Autodesk Inventor part; units mm, degrees
ref_plane "工作平面2" through (150, 0, 0) normal (-1, 0, 0) x (0, 0, 1)
ref_plane "YZ Plane" through (0, 0, 0) normal (1, 0, 0) x (0, 1, 0)
ref_plane "XZ Plane" through (0, 0, 0) normal (0, 1, 0) x (-1, 0, 0)
sketch "草圖1" plane through (0, 0, 0) normal (0, 0, 1) x (1, 0, 0)
  line L0 (0, 25) -> (300, 25)
  line L1 (300, 25) -> (300, 0)
  line L2 (300, 0) -> (0, 0)
  line L3 (0, 0) -> (0, 25)
  circle A0 centre (23, 17.5) radius 6.55
  circle A1 centre (277, 17.5) radius 2
  line L4 (16, 0) -> (24, 0)
  line L5 (24, 0) -> (24, -2.9)
  line L6 (24, -2.9) -> (16, -2.9)
  line L7 (16, -2.9) -> (16, 0)
  line L8 (276, 0) -> (284, 0)
  line L9 (284, 0) -> (284, -2.9)
  line L10 (284, -2.9) -> (276, -2.9)
  line L11 (276, -2.9) -> (276, 0)
  line L12 (0, 25) -> (5, 25)
  line L13 (5, 25) -> (5, 0)
  line L14 (5, 0) -> (0, 0)
  line L15 (0, 0) -> (0, 25)
  line L16 (300, 25) -> (295, 25)
  line L17 (295, 25) -> (295, 0)
  line L18 (295, 0) -> (300, 0)
  line L19 (300, 0) -> (300, 25)
  line L20 (24, -1.45) -> (276, -1.45) construction
  point P0 (16, -1.45)
  point P1 (284, -1.45)
  point P2 (284, 0)
  point P3 (24, 0)
  point P4 (150, -1.45)
  point P5 (150, 0)
  dimension "d0" = 300
  dimension "d1" = 25
  dimension "d2" = 7.5
  dimension "d3" = 13.1
  dimension "d4" = 23
  dimension "d5" = 23
  dimension "d6" = 7.5
  dimension "d7" = 4
  dimension "d12" = 8
  dimension "d13" = 2.9
  dimension "d14" = 8
  dimension "d30" = 5
  dimension "d31" = 5
  dimension "d32" = 252
extrude "擠出1" add sketch "草圖1" along normal blind 3 contours L0 L17 L2 L13 | L2 L5 L6 L7 | L9 L10 L11 L2
sketch "草圖2" plane through (0, 0, 3) normal (0, 0, 1) x (1, 0, 0)
  line L0 (10.5404, 25) -> (13.4864, 25.1544)
  line L1 (13.4864, 25.1544) -> (14.0097, 15.1681)
  line L2 (14.0097, 15.1681) -> (11.0638, 15.0137)
  line L3 (11.0638, 15.0137) -> (10.5404, 25)
  line L4 (295, 25) -> (5, 25)
  line L5 (16.048, 25) -> (29.13, 25.6856)
  line L6 (29.13, 25.6856) -> (30.1465, 6.2887)
  line L7 (30.1465, 6.2887) -> (17.0645, 5.6031)
  line L8 (17.0645, 5.6031) -> (16.048, 25)
  circle A0 centre (23, 17.5) radius 6.55
  line L9 (14.0097, 15.1681) -> (16.5562, 15.3016)
  line L10 (286.4135, 25.1544) -> (289.3595, 25)
  line L11 (289.3595, 25) -> (288.8361, 15.0137)
  line L12 (288.8361, 15.0137) -> (285.8901, 15.1681)
  line L13 (285.8901, 15.1681) -> (286.4135, 25.1544)
  line L14 (275.2453, 22.2337) -> (279.2399, 22.0243)
  line L15 (279.2399, 22.0243) -> (278.6818, 11.3762)
  line L16 (278.6818, 11.3762) -> (274.6873, 11.5855)
  line L17 (274.6873, 11.5855) -> (275.2453, 22.2337)
  circle A1 centre (277, 17.5) radius 2
  line L18 (285.8901, 15.1681) -> (278.8997, 15.5344)
  point P0 (0, 0)
  point P1 (300, 25)
  point P2 (0, 25)
  point P3 (286.4054, 25)
  point P4 (13.4945, 25)
  dimension "d16" = 2.95
  dimension "d18" = 10
  dimension "d19" = 87
  dimension "d20" = 87
  dimension "d22" = 87
  dimension "d23" = 87
  dimension "d24" = 2.95
  dimension "d25" = 10
  dimension "d33" = 9.1
  dimension "d34" = 9
extrude "擠出2" cut sketch "草圖2" against normal up to surface (3 mm away) contours L4 L11 L12 L13 | L4 L1 L2 L3
sketch "草圖7" plane through (0, 0, 3) normal (0, 0, 1) x (1, 0, 0)
  line L0 (64.4714, 28.6858) -> (65.4135, 10.7104)
  line L1 (65.4135, 10.7104) -> (7.493, 7.675)
  line L2 (7.493, 7.675) -> (6.5509, 25.6503)
  line L3 (6.5509, 25.6503) -> (64.4714, 28.6858)
  line L4 (13.4945, 25) -> (14.0097, 15.1681)
  circle A0 centre (23, 17.5) radius 6.55
  line L5 (285.8901, 15.1681) -> (286.4054, 25)
  line L6 (286.4054, 25) -> (13.4945, 25)
  line L7 (13.4945, 25) -> (14.0097, 15.1681)
  line L8 (14.0097, 15.1681) -> (11.0638, 15.0137)
  line L9 (11.0638, 15.0137) -> (10.5404, 25)
  line L10 (10.5404, 25) -> (5, 25)
  line L11 (5, 25) -> (5, 0)
  line L12 (5, 0) -> (16, 0)
  line L13 (16, 0) -> (16, -2.9)
  line L14 (16, -2.9) -> (24, -2.9)
  line L15 (24, -2.9) -> (24, 0)
  line L16 (24, 0) -> (276, 0)
  line L17 (276, 0) -> (276, -2.9)
  line L18 (276, -2.9) -> (284, -2.9)
  line L19 (284, -2.9) -> (284, 0)
  line L20 (284, 0) -> (295, 0)
  line L21 (295, 0) -> (295, 25)
  line L22 (295, 25) -> (289.3595, 25)
  line L23 (289.3595, 25) -> (288.8361, 15.0137)
  line L24 (288.8361, 15.0137) -> (285.8901, 15.1681)
  circle A1 centre (23, 17.5) radius 6.55
  circle A2 centre (277, 17.5) radius 2
  line L25 (13.4945, 25) -> (13.4414, 26.0114)
  line L26 (10.5404, 25) -> (11.0638, 15.0137)
  line L27 (10.5404, 25) -> (10.4955, 25.857)
  point P0 (0, 0)
  point P1 (64.6646, 25)
  point P2 (6.585, 25)
  dimension "d50" = 42
  dimension "d51" = 16
  dimension "d52" = 18
  dimension "d53" = 9
extrude "擠出5" add sketch "草圖7" against normal up to surface (3 mm away) contours L0 L6 L25 L3 | L27 L10 L2 L3
sketch "草圖9" plane through (0, 0, 3) normal (0, 0, 1) x (1, 0, 0)
  line L0 (10.4955, 25.857) -> (6.5509, 25.6503)
  line L1 (6.5509, 25.6503) -> (64.4714, 28.6858)
  line L2 (64.4714, 28.6858) -> (65.4135, 10.7104)
  line L3 (65.4135, 10.7104) -> (7.493, 7.675)
  line L4 (7.493, 7.675) -> (6.5509, 25.6503)
  circle A0 centre (58.1897, 24.3511) radius 2
  circle A1 centre (58.713, 14.3648) radius 2
  line L5 (58.1897, 24.3511) -> (58.713, 14.3648)
  line L6 (58.4513, 19.3579) -> (64.9424, 19.6981)
  circle A2 centre (23, 17.5) radius 6.55
  point P0 (0, 0)
  dimension "d60" = 18
  dimension "d64" = 4
  dimension "d66" = 6.5
  dimension "d67" = 10
extrude "擠出6" cut sketch "草圖9" against normal up to surface (3 mm away) contours A1 | A0
sketch "草圖11" plane through (0, 0, 3) normal (0, 0, 1) x (1, 0, 0)
  line L0 (16.45, 26.8556) -> (29.55, 26.8556)
  line L1 (29.55, 26.8556) -> (29.55, 17.5)
  line L2 (29.55, 17.5) -> (16.45, 17.5)
  line L3 (16.45, 17.5) -> (16.45, 26.8556)
  circle A0 centre (23, 17.5) radius 6.55
  line L4 (64.4714, 28.6858) -> (13.4414, 26.0114)
  point P0 (0, 0)
  dimension "d74" = 13.1
extrude "擠出7" cut sketch "草圖11" against normal blind 10 contours L0 L4 L3 | L1 A0 L3 L4 | L2 A0 picked at (21.0033, 19.0372)
ref_plane "工作平面2" through (150, 0, 0) normal (-1, 0, 0) x (0, 0, 1)
mirror "鏡射2" [suppressed]
sketch "草圖12" plane through (0, 0, 3) normal (0, 0, 1) x (1, 0, 0)
  arc A0 (279, 17.5) -> (279, 17.5) centre (277, 17.5) ccw
  line L0 (279, 17.5) -> (283.55, 17.5)
  circle A1 centre (277, 17.5) radius 6.55
  point P0 (0, 0)
extrude "擠出8" [suppressed]
sketch "草圖10" plane through (0, 0, 3) normal (0, 0, 1) x (1, 0, 0)
  line L0 (285.8901, 15.1681) -> (286.4054, 25)
  line L1 (286.4054, 25) -> (64.6646, 25)
  line L2 (14.0097, 15.1681) -> (11.0638, 15.0137)
  line L3 (6.585, 25) -> (5, 25)
  line L4 (5, 25) -> (5, 0)
  line L5 (5, 0) -> (16, 0)
  line L6 (16, 0) -> (16, -2.9)
  line L7 (16, -2.9) -> (24, -2.9)
  line L8 (24, -2.9) -> (24, 0)
  line L9 (24, 0) -> (276, 0)
  line L10 (276, 0) -> (276, -2.9)
  line L11 (276, -2.9) -> (284, -2.9)
  line L12 (284, -2.9) -> (284, 0)
  line L13 (284, 0) -> (295, 0)
  line L14 (295, 0) -> (295, 25)
  line L15 (295, 25) -> (289.3595, 25)
  line L16 (289.3595, 25) -> (288.8361, 15.0137)
  line L17 (288.8361, 15.0137) -> (285.8901, 15.1681)
  arc A0 (16.45, 17.5) -> (29.55, 17.5) centre (23, 17.5) ccw
  circle A1 centre (277, 17.5) radius 2
  line L18 (13.4414, 26.0114) -> (14.0097, 15.1681)
  line L19 (11.0638, 15.0137) -> (10.4955, 25.857)
  line L20 (64.6646, 25) -> (64.4714, 28.6858)
  line L21 (64.4714, 28.6858) -> (29.55, 26.8556)
  line L22 (10.4955, 25.857) -> (6.5509, 25.6503)
  line L23 (6.5509, 25.6503) -> (6.585, 25)
  line L24 (29.55, 26.8556) -> (29.55, 17.5)
  line L25 (16.45, 17.5) -> (16.45, 26.1691)
  line L26 (16.45, 26.1691) -> (13.4414, 26.0114)
  point P0 (0, 0)
equation "\"d20\" = d19"
equation "\"d22\" = d23"
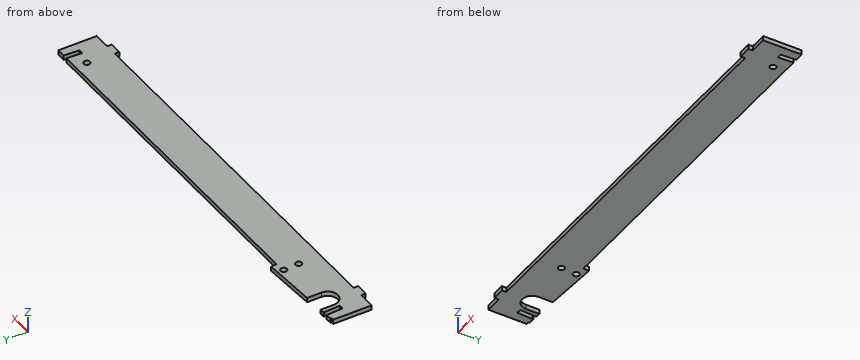
The model under review builds one solid part; all positions refer to its coordinate system, in mm. Coordinates: 2 decimals unless noted, no trailing zeros. Order: outer loops, then holes, each group sorted by start corner. A loop starts at its lowest first (then second) coordinate and runs counter-clockwise, first axis right, second up. Notation, with made-up numbers: (12.25, 25) -> (17.25, 25) arc R18 ccw to (17.25, 51) -> close; hole circle Ø4 at (68.25, 83). An arc over 180 degrees is marked (long way). Answer in a Markdown table with one row per item. Add a question column.
Item 1: We need section B-B on x = 232.5. Write out the cut boundary in (y, z), plus the area to 3 significant figures.
Item 2: Clearance check with flat-ended pins moving along their axes: pin 1 (0.9 mm diameter, centred on x = 292, z = 2, fed in from +Y); pin 2 (1.4 mm diameter, centred on y = -1, z = 1, fed in from -X); pin 3 (0.9 mm diameter, centred on x = 162.5, z = 1, fed in from -Y); pin 4 (2 mm diameter, centred on x = 216.5, y = 17, fed in from -Z). State where each tip first meets the part, or that it passes through.
Item 3: To check wall thickness, follow probe 1 along X at (y, z) = (24.5, 0.3); probe 2 along Y at (x, z) = (277, 2.05); probe 3 along X at (y, z) = (23, 1.3). State the ranges of each line that lie inside material, in increasing order.
Item 4: We need section C-C on x = 45. Write out the cut boundary in (y, z), plus the area to 3 significant figures.
Item 5: We need section A-A on z = 1.7. Give the number of separate pieces and of enclosed holes in the cut face, plus the area to 3 significant figures.
Final values:
| question | item | result |
|---|---|---|
| 1 | outline | (0, 0) -> (25, 0) -> (25, 3) -> (0, 3) -> close |
| 1 | area | 75.0 mm2 |
| 2 | pin 1 | stops at y = 25 |
| 2 | pin 2 | stops at x = 16 |
| 2 | pin 3 | stops at y = 0 |
| 2 | pin 4 | stops at z = 0 |
| 3 | probe 1 | x = 5 to 10.57, 13.52 to 16.45, 29.55 to 56.2, 60.18 to 286.38, 289.33 to 295 |
| 3 | probe 2 | y = -2.9 to 15.5, 19.5 to 25 |
| 3 | probe 3 | x = 5 to 10.65, 13.6 to 16.45, 29.55 to 56.72, 59.66 to 286.3, 289.25 to 295 |
| 4 | outline | (0, 0) -> (27.67, 0) -> (27.67, 3) -> (0, 3) -> close |
| 4 | area | 83.0 mm2 |
| 5 | separate pieces | 1 |
| 5 | enclosed holes | 3 |
| 5 | area | 7,140 mm2 |
